Geometry: final body of the model. Coordinates: model frame, mm. A direction names the side the tool comes from. Give positions to 0.01 mm unless a question says otherwise; leave off trailing zeros. Loops run counter-clockwise (first coordinate to the right, second up) from the corner with the lowest first, then second, coordinate; pieces in that order, holes last. Notation, with made-up numbers: (-0.5, 70.5) -> (56.5, 70.5) arc R24 ccw to (56.5, 99.5) -> close; hole circle Ø7 at (69.25, -4). An arc over 180 degrees is marked (long way). Answer in a Markdown table with one row per item. Add a question column.
from build123d import *

# Parameters (mm, degrees)
F1_DEPTH = 42
F3_DEPTH = 40
F5_DEPTH = 10
F6_T     = -1.5
F7_R     = 1


# Not quite as in the source:
# - a shell that OpenCascade refuses in one call is made with other operations: the cavity is built on its own and cut out


with BuildPart() as f1:
    # F0 (on Top) → F1 (new body)
    with BuildSketch(Plane.XY):
        Polygon((-33.486315613, 29), (-16.7431578065, 0), (-33.486315613, -29), (-16.7431578065, -58), (16.7431578065, -58), (33.486315613, -29), (16.7431578065, 0), (33.486315613, 29), (16.7431578065, 58), (-16.7431578065, 58), align=None)
    extrude(amount=F1_DEPTH)

    # F2 (on face) → F3 (cut)
    with BuildSketch(Plane.XY.offset(42)):
        Polygon((15.7327948354, -1.75), (0, -1.75), (-15.7327948354, -1.75), (-31.4655896708, -29), (-15.7327948354, -56.25), (15.7327948354, -56.25), (31.4655896708, -29), align=None)
        Polygon((-15.7327948354, 1.75), (0, 1.75), (15.7327948354, 1.75), (31.4655896708, 29), (15.7327948354, 56.25), (-15.7327948354, 56.25), (-31.4655896708, 29), align=None)
    extrude(amount=-F3_DEPTH, mode=Mode.SUBTRACT)

    # F4 (on face) → F5 (join)
    with BuildSketch(Plane.XY.offset(42)):
        Polygon((32.4877562844, 10.1850116625), (20.7271178342, 10.1850116625), (14.8467986091, 0), (20.7271178342, -10.1850116625), (32.4877562844, -10.1850116625), (38.3680755094, 0), align=None)
    extrude(amount=-F5_DEPTH)

    # F6: a shell. OpenCascade refuses it in one call, so the cavity is built on its own and cut out:
    # the body offset inwards by the wall thickness, plus a prism from it out through each open face.
    f6_core = offset(f1.part, amount=F6_T, kind=Kind.INTERSECTION, mode=Mode.PRIVATE)
    f6_exits = [f6_core.faces().sort_by_distance(p)[0] for p in [
        (26.515913, 0, 33.5),
    ]]
    add(f6_core, mode=Mode.SUBTRACT)
    extrude(f6_exits, amount=-F6_T, mode=Mode.SUBTRACT)

    # F7
    f7_edges = [f1.edges().sort_by_distance(p)[0] for p in [
        (-33.486316, -29, 21),
        (-16.743158, 0, 21),
        (-33.486316, 29, 21),
        (-16.743158, 58, 21),
        (-16.743158, -58, 21),
        (16.743158, -58, 21),
        (33.486316, -29, 21),
        (16.743158, 0, 16),
        (33.486316, 29, 21),
        (16.743158, 58, 21),
        (-31.46559, 29, 22),
        (-15.732795, 56.25, 22),
        (15.732795, 56.25, 22),
        (31.46559, 29, 22),
        (15.732795, 1.75, 22),
        (-15.732795, 1.75, 22),
        (-31.46559, -29, 22),
        (-15.732795, -1.75, 22),
        (15.732795, -1.75, 22),
        (31.46559, -29, 22),
        (15.732795, -56.25, 22),
        (-15.732795, -56.25, 22),
        (0, 1.75, 2),
        (23.599192, 15.375, 2),
        (23.599192, 42.625, 2),
        (0, 56.25, 2),
        (-23.599192, 42.625, 2),
        (-23.599192, 15.375, 2),
        (0, -1.75, 2),
        (-23.599192, -15.375, 2),
        (-23.599192, -42.625, 2),
        (0, -56.25, 2),
        (23.599192, -42.625, 2),
        (23.599192, -15.375, 2),
        (-25.114737, 14.5, 0),
        (-25.114737, -14.5, 0),
        (-25.114737, -43.5, 0),
        (0, -58, 0),
        (25.114737, -43.5, 0),
        (25.114737, -14.5, 0),
        (25.114737, 14.5, 0),
        (25.114737, 43.5, 0),
        (0, 58, 0),
        (-25.114737, 43.5, 0),
        (22.623477, 10.185012, 37),
        (32.487756, 10.185012, 37),
        (38.368076, 0, 37),
        (32.487756, -10.185012, 37),
        (22.623477, -10.185012, 37),
    ]]
    fillet(f7_edges, radius=F7_R)


solid = f1.part
(1) Pin query (flat end, axial travel): pin 1 Ø8 at (x, y) = (-8.5, 5) entering from +Z; pin 2 Ø7 at (x, z) = (27.5, 36.5) entering from -Y; pin 3 Ø10 at (x, z) = (30, 16.5) entering from -Y; pin 4 Ø2.5 at (x, z) = (28, 38.5) entering from -Y. Return the tip coordinate at first contact, or that it passes through.
(2) Reachability of faces 1 (the flat face through (-25, -14.3, 21.2)), 2 (the flat face through (25.23, -14.7, 21.21)), 3 (the flat face through (0, 0.25, 21)), 4 (the flat face through (0, -56.25, 23)) from +Z, -Z, +X, -X, +Y, -Y: full face, straight path, thin tool, end or side. Return the list, or none.
(3) Draft query along X for faces 5 (the cylindrical face through (24.755, -14.447, 0.301)), 6 (the cylindrical face through (-23.458, -15.701, 2.301)), 7 (the cylindrical face through (-24.755, 14.447, 0.301)). Return one class per face: +X half, -X half, draft (parallel to the pull), parting line (faces both ways), or undercut.
(4) Material intervals for line 1 along Y through (x, z) = (-9, 21); line 2 along Y through (x, z) = (29.5, 33), sorted ascending. Write a range as from..to.
(5) Cut plane B-B on z = 19.5. State how many separate pieces and enclosed holes the cut face has, then the cut area to 3 significant figures.
(6) Cut plane A-A on x = 3. Return the cut outline in (y, z), then the cut area to 3 significant figures.
Answer list:
| question | item | result |
|---|---|---|
| 1 | pin 1 | stops at z = 42 |
| 1 | pin 2 | stops at y = -45.43 |
| 1 | pin 3 | stops at y = -43.7 |
| 1 | pin 4 | stops at y = -40.67 |
| 2 | face 1 | +Z, -Z, -X |
| 2 | face 2 | -Z, +X |
| 2 | face 3 | none |
| 2 | face 4 | +Z |
| 3 | face 5 | +X half |
| 3 | face 6 | undercut |
| 3 | face 7 | -X half |
| 4 | line 1 | y = -58..-56.25, -1.75..-0.25, 0.25..1.75, 56.25..58 |
| 4 | line 2 | y = -35.9..-32.4, -25.6..-22.1, -10.19..-8.69, 8.69..10.19, 22.1..25.6, 32.4..35.9 |
| 5 | separate pieces | 1 |
| 5 | enclosed holes | 3 |
| 5 | area | 667 mm² |
| 6 | outline | (-58, 1) arc R1 ccw to (-57, 0) -> (57, 0) arc R1 ccw to (58, 1) -> (58, 42) -> (56.25, 42) -> (56.25, 3) arc R1 cw to (55.25, 2) -> (2.75, 2) arc R1 cw to (1.75, 3) -> (1.75, 42) -> (-1.75, 42) -> (-1.75, 3) arc R1 cw to (-2.75, 2) -> (-55.25, 2) arc R1 cw to (-56.25, 3) -> (-56.25, 42) -> (-58, 42) -> close; hole (-0.25, 1.5) -> (0.25, 1.5) -> (0.25, 40.5) -> (-0.25, 40.5) -> close |
| 6 | area | 493 mm² |
